Could you check a few things on this drawing? It's one solid part, dimensions in mm from its lowest x, y, z. Give positions to 0.01 mm unless a question says otherwise; leave off trailing zeros. Loops run counter-clockwise (first coordinate to the right, second up) from the corner with the lowest first, then second, coordinate; pieces in that order, holes last. Notation, with made-up numbers: M 71,-21 L 113,-21 A32 cw 113,11 Z; hole C 6.25,24 d5. An arc over 180 degrees is marked long. Return JSON: item names as keys, results as strings. Group by question number.
1. If we section it at A-A (z = 1.75): Write out the boundary of the cut face in (x, y), plus the area to 3 significant figures.
2. Please list where these lines run through material, in increasing order: line 1 (Y direction, x = 54, z = 1.85); line 2 (X direction, y = 2, z = 1.7).
3. If we section it at C-C (x = 25.5): Write out the boundary of the cut face in (y, z), plus the area to 3 significant figures.
4. If we section it at B-B (y = 4): Write out the boundary of the cut face in (x, z), plus the area to 3 significant figures.
5. For pin 1 (1.5 mm diameter, centred on y = 38, z = 1.5, fed in from -X); pin 2 (1.5 mm diameter, centred on y = 39, z = 2, fed in from +X); pin 3 (0.9 mm diameter, centred on x = 126, z = 1, fed in from +Y), each with a flat end and sliding along its axis, tell me the tip position at first contact or that it passes through.
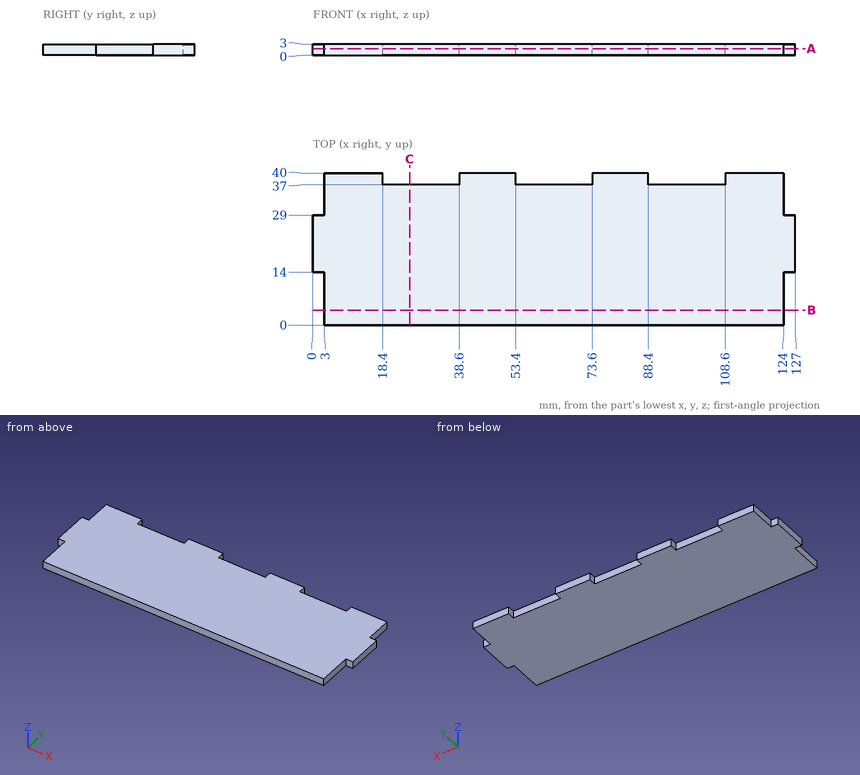
Answer:
{
 "1": {"outline": "M 0,14 L 3,14 L 3,0 L 124,0 L 124,14 L 127,14 L 127,29 L 124,29 L 124,40 L 108.6,40 L 108.6,37 L 88.4,37 L 88.4,40 L 73.6,40 L 73.6,37 L 53.4,37 L 53.4,40 L 38.6,40 L 38.6,37 L 18.4,37 L 18.4,40 L 3,40 L 3,29 L 0,29 Z", "area": "4,750 mm²"},
 "2": {"line 1": "y = 0 to 37", "line 2": "x = 3 to 124"},
 "3": {"outline": "M 0,0 L 37,0 L 37,3 L 0,3 Z", "area": "111 mm²"},
 "4": {"outline": "M 3,0 L 124,0 L 124,3 L 3,3 Z", "area": "363 mm²"},
 "5": {"pin 1": "stops at x = 3", "pin 2": "stops at x = 124", "pin 3": "stops at y = 29"}
}
